The drawing under review shows one solid part. Ordinate dimensions are in mm from its lowest x, y, z. Coordinates: 2 decimals unless noted, no trailing zeros. Loops run counter-clockwise (first coordinate to the right, second up) from the corner with the lowest first, then second, coordinate; pieces in that order, holes last. Notation, with made-up numbers: (-6.5, 46) -> (29.5, 46) arc R9 ccw to (29.5, 58) -> close; hole circle Ø1 at (47.5, -24.75). An arc over 180 degrees is marked (long way). Use a Markdown table: item, result.
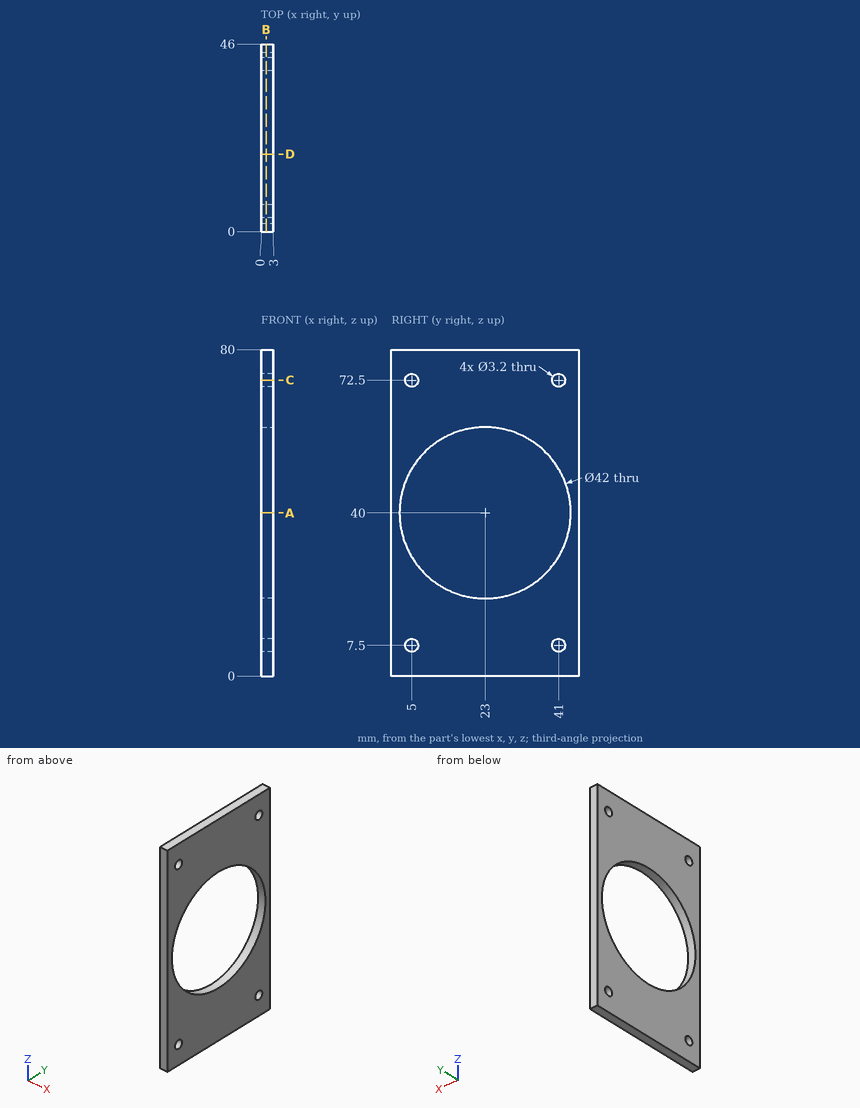
(1) Take a section at B-B on x = 1.25. Write out the cut boundary in (y, z), plus the area to 3 significant figures.
Found:
| item | result |
|---|---|
| outline | (0, 0) -> (46, 0) -> (46, 80) -> (0, 80) -> close; hole circle Ø42 at (23, 40); hole circle Ø3.2 at (5, 7.5); hole circle Ø3.2 at (5, 72.5); hole circle Ø3.2 at (41, 7.5); hole circle Ø3.2 at (41, 72.5) |
| area | 2,260 mm^2 |
(2) Take a section at D-D on y = 19. Write out the cut boundary in (x, z), plus the area to 3 significant figures.
Found:
| item | result |
|---|---|
| outline | (0, 0) -> (3, 0) -> (3, 19.38) -> (0, 19.38) -> close; (0, 60.62) -> (3, 60.62) -> (3, 80) -> (0, 80) -> close |
| area | 116 mm^2 |
(3) For line 1 along Y through (x, z) = (1, 7.5); line 2 along Y through (x, z) = (1.3, 40); line 3 along Z through (x, y) = (1, 41), list the stretches that pass through material, from the lowest coordinate up.
Found:
| item | result |
|---|---|
| line 1 | y = 0 to 3.4, 6.6 to 39.4, 42.6 to 46 |
| line 2 | y = 0 to 2, 44 to 46 |
| line 3 | z = 0 to 5.9, 9.1 to 29.18, 50.82 to 70.9, 74.1 to 80 |
(4) Take a section at C-C on z = 72.5. Write out the cut boundary in (x, y).
Found:
| item | result |
|---|---|
| outline | (0, 0) -> (3, 0) -> (3, 3.4) -> (0, 3.4) -> close; (0, 6.6) -> (3, 6.6) -> (3, 39.4) -> (0, 39.4) -> close; (0, 42.6) -> (3, 42.6) -> (3, 46) -> (0, 46) -> close |
(5) Take a section at A-A on z = 40. Write out the cut boundary in (x, y), plus the area to 3 significant figures.
Found:
| item | result |
|---|---|
| outline | (0, 0) -> (3, 0) -> (3, 2) -> (0, 2) -> close; (0, 44) -> (3, 44) -> (3, 46) -> (0, 46) -> close |
| area | 12.0 mm^2 |
(6) For pin 1 Ø3 at (y, z) = (41, 72.5) entering from -X, flat-tipped, find the tip position at first contact; note if it passes through.
Found:
| item | result |
|---|---|
| pin 1 | passes through |
